```python
from build123d import *

# Parameters (mm, degrees)
F0_R      = 38.6812763638
F1_DEPTH  = 5.08
F2_R      = 4.0500019282
F3_DEPTH  = 76.2
F4_W      = 3.1792044174
F4_H      = 16.6880693287
F4_W_2    = 18.8102982938
F4_H_2    = 2.3871629965
F4_W_3    = 2.9142722487
F4_H_3    = 14.3064234871
F5_DEPTH  = 2.54
F6_R      = 1.27
F8_R      = 6.6885556935
F8_R_2    = 5.9347433367
F8_R_3    = 6.3640715152
F8_R_4    = 6.1622808629
F9_DEPTH  = 7.62
F11_DEPTH = 7.621


# Not quite as in the source:
# - a fillet or chamfer that OpenCascade refuses, or shapes differently, is made with other operations: its cross-section is extruded or revolved along the edge and cut away or added


with BuildPart() as f1:
    # F0 (on Top) → F1 (new body)
    with BuildSketch(Plane.XY):
        Circle(F0_R)
    extrude(amount=F1_DEPTH)

    # F2 (on face) → F3 (join)
    with BuildSketch(Plane(origin=(0, 0, 0), x_dir=(1, 0, 0), z_dir=(0, 0, -1))):
        Circle(F2_R)
    extrude(amount=F3_DEPTH)

    # F4 (on face) → F5 (join)
    with BuildSketch(Plane(origin=(0, 0, -76.2), x_dir=(1, 0, 0), z_dir=(0, 0, -1))):
        with Locations((1.5896022087, 8.3440346643)):
            Rectangle(F4_W, F4_H)
        Polygon((3.1792044174, 0), (0, 0), (0, -2.3871629965), (2.9142722487, -2.3871629965), (20.6648353487, -2.3871629965), (20.6648353487, 0), align=None)
        with Locations((-9.4051491469, -1.1935814982)):
            Rectangle(F4_W_2, F4_H_2)
        with Locations((1.4571361244, -9.54037474)):
            Rectangle(F4_W_3, F4_H_3)
    extrude(amount=F5_DEPTH)

    # F6
    f6_edges = [f1.edges().sort_by_distance(p)[0] for p in [
        (-38.681276, 0, 0),
    ]]
    fillet(f6_edges, radius=F6_R)

    # F7: fillet of radius 5.08 on 1 edges, made by hand

    # F7_s1 → F7_t2 (revolve, cut)
    with BuildSketch(Plane.XZ):
        with BuildLine():
            ThreePointArc((38.6812763638, 1.27), (36.8734394874, 4.0160926284), (33.7625875141, 5.08))
            Line((33.7625875141, 5.08), (33.7625875141, 5.1816))
            Line((33.7625875141, 5.1816), (38.6812763638, 5.1816))
            Line((38.6812763638, 5.1816), (38.7828763638, 5.08))
            ThreePointArc((38.7828763638, 5.08), (38.7828763638, 3.175), (38.7796501408, 1.2954))
            Line((38.7796501408, 1.2954), (38.6812763638, 1.27))
        make_face()
    revolve(axis=Axis((0, 0, 5.08), (0, 0, 1)), mode=Mode.SUBTRACT)

    # F8 (on face) → F9 (join)
    with BuildSketch(Plane(origin=(0, 0, -78.74), x_dir=(1, 0, 0), z_dir=(0, 0, -1))):
        with Locations((20.6648353487, 0)):
            Circle(F8_R)
        with Locations((-18.8102982938, 0)):
            Circle(F8_R_2)
        with Locations((2.9142722487, -16.6935864836)):
            Circle(F8_R_3)
        with Locations((3.1792044174, 16.6880693287)):
            Circle(F8_R_4)
    extrude(amount=F9_DEPTH)

    # F10 (on face) → F11 (cut, through all)
    with BuildSketch(Plane.XY.offset(-78.74)):
        Polygon((1.4149318504, 22.8785185463), (8.4209625868, 13.5033250881), (25.2221585853, 26.6414508232), (18.2112082839, 35.6629639864), (10.4142271803, 29.6036426698), align=None)
    extrude(amount=-F11_DEPTH, mode=Mode.SUBTRACT)


solid = f1.part
```
Read the model definition and answer for the solid it produces. Units are mm, in the model's axes. A direction names the side the tool comes from. Give positions to 0.01 mm unless a question says otherwise; leave off trailing zeros. Order: outer loops, then holes, each group sorted by start corner. A loop starts at its lowest first (then second) coordinate and runs counter-clockwise, first axis right, second up. Notation, with made-up numbers: (79, 36.25) -> (109, 36.25) arc R24 cw to (109, 73.25) -> close; hole circle Ø3 at (29.25, -14.5). An arc over 180 degrees is marked (long way). One line per item, written item: value. Start each with the question number.
(1) A tool of negligible diameter and unlimited length cuts with its end or side. For faces 4 (the flat face through (-10, 2.387, -77)), 5 (the flat face through (1, 16.694, -77)), 6 (the flat face through (-10, 0, -77)), 7 (the cylindrical face through (-2.076, 12.745, -82.497)), from which of +Z, -Z, +X, -X, +Y, -Y can it reach the whole face along a straight path? Write none if from no direction.
(2) For a pull along Z with two mould halves and no side action, classify faces 1 (the flat face through (0, 0, 5.08)), 2 (the flat face through (2, -16.688, -77)), 3 (the flat face through (1, 17, -86.36)) as released by +Z, released by -Z, zero draft, split by the parting line, or undercut.
(3) Straight lines are drawn through the part: L1, parallel to Y at x = -10, z = -78; L2, parallel to Z at x = 26.5, y = -4; L3, parallel to X at y = -5.5, z = -76.5. For each, find the intervals that lie inside material, in ascending order.
(4) The part is cut by section A-A (z = -39). Determine the outline of the cut face in (x, y).
(5) Flat-ended cylindrical pins translate along their axes: P1, Ø3, axis at x = -23, y = -21.5, coming from the -Z side; P2, Ø6.5, axis at x = 2, y = -0.5, coming from the -Z side; P3, Ø5, axis at x = -26.5, y = -30.5, coming from the -Z side. Find the tip coordinate at first contact, or state that the pin passes through.
Taken from the geometry:
1. face 4: -X, +Y
1. face 5: +X, -X, +Y
1. face 6: -X, -Y
1. face 7: -Z
2. face 1: released by +Z
2. face 2: undercut
2. face 3: released by -Z
3. L1: 0 to 2.39
3. L2: 0 to 5.08
3. L3: 0 to 3.18
4. outline: circle Ø8.1 at (0, 0)
5. P1: z = 0
5. P2: z = -78.74
5. P3: z = 0.1
